from build123d import *

# Parameters (mm, degrees)
BOSS_EXTRUDE1_DEPTH = 10


with BuildPart() as part:
    # Sketch1 → Boss-Extrude1 (new body)
    with BuildSketch(Plane.XY):
        Polygon((40, 107), (23, 113), (15, 120), (15, 170), (31.055768347, 170), (46.225269869, 166.291261256), (62.793848643, 155.971389715), (77.033804463, 155.971389715), (77.033804463, 170.971389715), (75.085424996, 180.171389715), (60, 191.5), (39.787088413, 198), (0, 200), (-39.787088413, 198), (-60, 191.5), (-75.085424996, 180.171389715), (-77.033804463, 170.971389715), (-77.033804463, 155.971389715), (-62.793848643, 155.971389715), (-46.225269869, 166.291261256), (-31.055768347, 170), (-15, 170), (-15, 120), (-23, 113), (-40, 107), (-60, 25), (-85, 25), (-85, 0), (85, 0), (85, 25), (60, 25), align=None)
    extrude(amount=BOSS_EXTRUDE1_DEPTH)


solid = part.part
Work out the finished part from the listing and answer in its coordinate system (mm). A direction names the side the tool comes from. Coordinates: 2 decimals unless noted, no trailing zeros. Write each loop counter-clockwise with the first axis right and the second up, starting at its lowest first coordinate (ties: lowest second). Pieces come first, ordered by that corner, then holes. Notation, with made-up numbers: M -31.75,56.25 L 17.25,56.25 A28 ccw 17.25,89.25 Z; hole C 41.25,60.5 d2. An arc over 180 degrees is marked long. Write item = value, one per line.
1. The part is cut by section C-C (y = 40). Determine the outline of the cut face in (x, z).
Solution:
outline = M -56.34,0 L 56.34,0 L 56.34,10 L -56.34,10 Z
2. The part is cut by section B-B (y = 130.5). Determine the outline of the cut face in (x, z).
Solution:
outline = M -15,0 L 15,0 L 15,10 L -15,10 Z
3. For faces 1 (the face through (-54.626, 161.059, 4.93)), 2 (the face through (-31.381, 110.042, 4.93)), 3 (the face through (-77.034, 164, 5)), 4 (the face through (19.06, 116.45, 4.93)), determine the directions among +Z, -Z, +X, -X, +Y, -Y from which every point of the face is accessible in a straight line to the end or side of a thin tool.
Solution:
face_1 = +Z, -Z
face_2 = +Z, -Z, -X
face_3 = +Z, -Z, -X, +Y
face_4 = +Z, -Z, +X
4. Flat-ended cylindrical pins translate along their axes: pin 1 (5 mm diameter, centred on y = 157.5, z = 4, fed in from +X); pin 2 (3 mm diameter, centred on x = 60, z = 8.5, fed in from +Y); pin 3 (1.5 mm diameter, centred on y = 90.5, z = 6.5, fed in from -X). Find the tip coordinate at first contact, or state that the pin passes through.
Solution:
pin_1 = 77.03
pin_2 = 191.98
pin_3 = -44.21
5. Straight lines are drawn through the part: line 1 (X direction, y = 138, z = 3.5); line 2 (Y direction, x = 73, z = 5.25); line 3 (Y direction, x = 30.5, z = 5.75). For each, find the intervals that lie inside material, in ascending order. Write a range as from..to.
Solution:
line_1 = -15..15
line_2 = 0..25, 155.97..181.74
line_3 = 0..110.35, 170..198.47
6. Determine the mould class of faces 5 (the face through (-15, 145, 5)), 6 (the face through (-1, 101, 0)), 7 (the face through (85, 12, 5)), 8 (the face through (-38.75, 168.12, 4.93)) for opening direction X: released by +X, released by -X, zero draft, split by the parting line, or undercut.
Solution:
face_5 = undercut
face_6 = zero draft
face_7 = released by +X
face_8 = undercut
